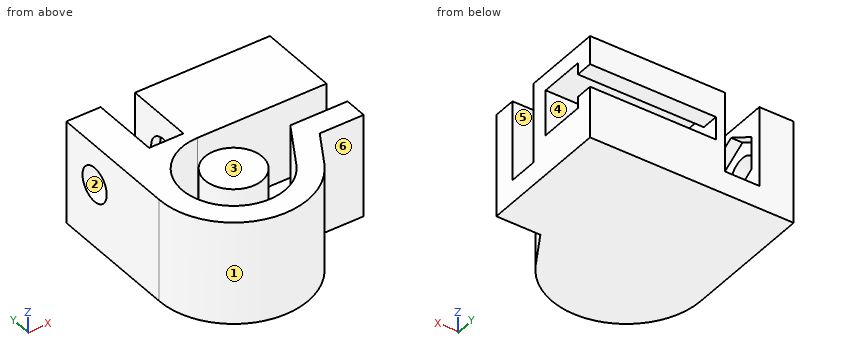
from build123d import *

# Parameters (mm, degrees)
ESBO_O1_R                  = 2.5
RESSALTO_EXTRUS_O1_DEPTH   = 7
RESSALTO_EXTRUS_O1_2_DEPTH = 7
CORTE_EXTRUS_O1_DEPTH      = 1
CORTE_EXTRUS_O2_DEPTH      = 21.752652218
CORTE_EXTRUS_O2_DEPTH_BACK = 21.752652218
ESBO_O4_R                  = 1.5
CORTE_EXTRUS_O3_DEPTH      = 11
RESSALTO_EXTRUS_O5_START   = -7
ESBO_O6_W                  = 3
ESBO_O6_H                  = 6
RESSALTO_EXTRUS_O5_DEPTH   = 2


with BuildPart() as part:
    # Esbo_o1 → Ressalto-extrus_o1 (new body)
    with BuildSketch(Plane.XY):
        Circle(ESBO_O1_R)
    extrude(amount=RESSALTO_EXTRUS_O1_DEPTH)



with BuildPart() as body_2:
    # Esbo_o1 → Ressalto-extrus_o1 2 (new body)
    with BuildSketch(Plane.XY):
        with BuildLine():
            ThreePointArc((0, 4.5), (-3.897114317, -2.25), (3.897114317, -2.25))
            Line((3.897114317, -2.25), (6.293117934, 1.9))
            Line((6.293117934, 1.9), (11.293117934, 1.9))
            Line((11.293117934, 1.9), (11.293117934, -0.1))
            Line((11.293117934, -0.1), (7.447818473, -0.1))
            Line((7.447818473, -0.1), (5.629165125, -3.25))
            ThreePointArc((5.629165125, -3.25), (-1.682323793, -6.278517871), (-6.5, 0))
            Line((-6.5, 0), (-6.5, 11.5))
            Line((-6.5, 11.5), (-3.5, 11.5))
            Line((-3.5, 11.5), (-3.5, 5.5))
            Line((-3.5, 5.5), (-0.5, 5.5))
            Line((-0.5, 5.5), (-0.5, 11.5))
            Line((-0.5, 11.5), (11.293117934, 11.5))
            Line((11.293117934, 11.5), (11.293117934, 6.5))
            Line((11.293117934, 6.5), (11.293117934, 4.5))
            Line((11.293117934, 4.5), (0, 4.5))
        make_face()
    extrude(amount=RESSALTO_EXTRUS_O1_2_DEPTH)

    # Esbo_o2 → Corte-extrus_o1 (cut)
    with BuildSketch(Plane(origin=(-3.5, 0, 0), x_dir=(0, 0, -1), z_dir=(1, 0, 0))):
        Polygon((-0.613248654, 8), (-2.056624327, 10.5), (-4.943375673, 10.5), (-6.386751346, 8), (-4.943375673, 5.5), (-2.056624327, 5.5), align=None)
    extrude(amount=-CORTE_EXTRUS_O1_DEPTH, mode=Mode.SUBTRACT)

    # Esbo_o4 → Corte-extrus_o2 (cut, two sides: drawn at the far end of the back side and taken through both)
    with BuildSketch(Plane(origin=(-4.5, 0, 0), x_dir=(0, 0, -1), z_dir=(1, 0, 0)).offset(-CORTE_EXTRUS_O2_DEPTH_BACK)):
        with Locations(Location((-3.5, 8, 0), (0, 0, 90))):
            Circle(ESBO_O4_R)
    extrude(amount=CORTE_EXTRUS_O2_DEPTH + CORTE_EXTRUS_O2_DEPTH_BACK, mode=Mode.SUBTRACT)

    # Esbo_o5 → Corte-extrus_o3 (cut)
    with BuildSketch(Plane(origin=(11.293117934, 0, 0), x_dir=(0, 0, -1), z_dir=(1, 0, 0))):
        Polygon((-5.5, 10), (-4.5, 10), (-4.5, 11.5), (-2.5, 11.5), (-2.5, 10), (-1.5, 10), (-1.5, 6), (-5.5, 6), align=None)
    extrude(amount=-CORTE_EXTRUS_O3_DEPTH, mode=Mode.SUBTRACT)


with BuildPart() as part_1:
    add(part.part)

    add(body_2.part)  # Ressalto-extrus_o5 merges body 2
    # Esbo_o6 → Ressalto-extrus_o5 (add)
    with BuildSketch(Plane.XY.offset(7).offset(RESSALTO_EXTRUS_O5_START)):
        with BuildLine():
            Line((11.293117934, 1.9), (11.293117934, 4.5))
            Line((11.293117934, 4.5), (0, 4.5))
            ThreePointArc((0, 4.5), (-3.897114317, -2.25), (3.897114317, -2.25))
            Line((3.897114317, -2.25), (6.293117934, 1.9))
            Line((6.293117934, 1.9), (11.293117934, 1.9))
        make_face()
        with BuildLine():
            ThreePointArc((3.897114317, -2.25), (-3.897114317, -2.25), (0, 4.5))
            Line((0, 4.5), (11.293117934, 4.5))
            Line((11.293117934, 4.5), (11.293117934, 11.5))
            Line((11.293117934, 11.5), (-0.5, 11.5))
            Line((-0.5, 11.5), (-0.5, 5.5))
            Line((-0.5, 5.5), (-3.5, 5.5))
            Line((-3.5, 5.5), (-3.5, 11.5))
            Line((-3.5, 11.5), (-6.5, 11.5))
            Line((-6.5, 11.5), (-6.5, 0))
            ThreePointArc((-6.5, 0), (-1.682323793, -6.278517871), (5.629165125, -3.25))
            Line((5.629165125, -3.25), (7.447818473, -0.1))
            Line((7.447818473, -0.1), (11.293117934, -0.1))
            Line((11.293117934, -0.1), (11.293117934, 1.9))
            Line((11.293117934, 1.9), (6.293117934, 1.9))
            Line((6.293117934, 1.9), (3.897114317, -2.25))
        make_face()
        with Locations((-2, 8.5)):
            Rectangle(ESBO_O6_W, ESBO_O6_H)
    extrude(amount=-RESSALTO_EXTRUS_O5_DEPTH)


solid = part_1.part
Model file for the job. Use its own axes, mm. Face numbers are marked on the shaded views. A direction names the side the tool comes from. Give positions to 0.01 mm unless a question says otherwise; leave off trailing zeros. Write each loop counter-clockwise with the first axis right and the second up, starting at its lowest first coordinate (ties: lowest second). Pieces come first, ordered by that corner, then holes. Notation, with made-up numbers: (-14, 37.5) -> (4, 37.5) arc R25 ccw to (4, 71.5) -> close; hole circle Ø10 at (70.5, 65.25). An arc over 180 degrees is marked (long way). Write item = value, one per line.
(1) Flat gauge pins, fed straight in: P1, Ø2.5, axis at y = 8, z = 3.5, coming from the -X side; P2, Ø2.5, axis at x = -2, y = 9, coming from the +Z side; P3, Ø1.9, axis at x = 10, z = 1, coming from the -Y side. Where does each tip first touch, or does it go through?
Determined:
P1 = through
P2 = 0
P3 = -0.1
(2) Slice it at A-A, the plane z = 3.5. Give the cut face in (x, y).
Determined:
outline = (-6.5, 0) arc R6.5 ccw to (5.63, -3.25) -> (7.45, -0.1) -> (11.29, -0.1) -> (11.29, 1.9) -> (6.29, 1.9) -> (3.9, -2.25) arc R4.5 cw (long way) to (0, 4.5) -> (11.29, 4.5) -> (11.29, 6) -> (0.29, 6) -> (0.29, 6.5) -> (-0.5, 6.5) -> (-0.5, 5.5) -> (-4.5, 5.5) -> (-4.5, 6.5) -> (-6.5, 6.5) -> close; (-6.5, 9.5) -> (-4.5, 9.5) -> (-4.5, 10.5) -> (-3.5, 10.5) -> (-3.5, 11.5) -> (-6.5, 11.5) -> close; circle Ø5 at (0, 0); (-0.5, 9.5) -> (0.29, 9.5) -> (0.29, 11.5) -> (-0.5, 11.5) -> close
(3) Tool access for the marked faces 4, 5 and 6: list every direction of +Z, -Z, +X, -X, +Y, -Y with a clear straight run to the whole face (end or side of a thin tool).
Determined:
face_4 = +X
face_5 = +Z, +X
face_6 = +Z, -Z, +X, -Y
(4) Slice it at C-C, the plane y = 0.5. Give the cut face in (x, z).
Determined:
outline = (-6.5, -2) -> (11.29, -2) -> (11.29, 7) -> (5.48, 7) -> (5.48, 0) -> (2.45, 0) -> (2.45, 7) -> (-2.45, 7) -> (-2.45, 0) -> (-4.47, 0) -> (-4.47, 7) -> (-6.5, 7) -> close
(5) Probe line 1 along Y through (x, z) = (-0.1, 3.5); line 2 along Z through (x, y) = (-6, 8); line 3 along Z through (x, y) = (7.5, 8). List the from-to ranges inside material, lowest first.
Determined:
line_1 = -6.5 to -4.5, -2.5 to 2.5, 4.5 to 6.5, 9.5 to 11.5
line_2 = -2 to 2, 5 to 7
line_3 = -2 to 1.5, 5.5 to 7
(6) Slice it at D-D, the plane z = -0.5. Give the cut face in (x, y).
Determined:
outline = (-6.5, 0) arc R6.5 ccw to (5.63, -3.25) -> (7.45, -0.1) -> (11.29, -0.1) -> (11.29, 11.5) -> (-6.5, 11.5) -> close
(7) Mould opens along Z. For the marked faces 1, 2 and 3 say: released by +Z, released by -Z, zero draft, split by the parting line, or undercut.
Determined:
face_1 = zero draft
face_2 = undercut
face_3 = released by +Z
(8) Slice it at B-B, the plane x = 8.75. Give the cut face in (y, z), then the cut area to 3 significant figures.
Determined:
outline = (-0.1, -2) -> (11.5, -2) -> (11.5, 2.5) -> (10, 2.5) -> (10, 1.5) -> (6, 1.5) -> (6, 5.5) -> (10, 5.5) -> (10, 4.5) -> (11.5, 4.5) -> (11.5, 7) -> (4.5, 7) -> (4.5, 0) -> (1.9, 0) -> (1.9, 7) -> (-0.1, 7) -> close
area = 67.2 mm2
